Geometry check sheet. Reference: the model listing, model coordinates, mm. Round coordinates to 2 decimals unless told otherwise and drop trailing zeros. Write each loop counter-clockwise with the first axis right and the second up, starting at its lowest first coordinate (ties: lowest second). Pieces come first, ordered by that corner, then holes. Notation, with made-up numbers: M 48.25,13.5 L 72.25,13.5 A20 ccw 72.25,45.5 Z; hole C -11.75,-33.5 d2. An arc over 180 degrees is marked long. One line per item, written item: value. Start each with the question number.
1. Section check C-C (x = 3). Record the boundary of the cut face in (y, z) (1 decimal), and give its area (3 significant figures).
2. Scan lines: probe 1 along X at (y, z) = (45, 0.75); probe 2 along X at (y, z) = (49, 4.25); probe 3 along X at (y, z) = (32, -2). Record each from-to range of solid material in increasing order. Write a range as [from, to].
3. Section check A-A (z = 0.5). Record the boundary of the cut face in (x, y) (1 decimal).
4. Section check B-B (y = -1.5). Record the boundary of the cut face in (x, z), and give its area (3 significant figures).
5. Depth check by flat-ended pin: P1, Ø1.8, axis at x = -3.18, y = 49.21, coming from the -Z side; P2, Ø1, axis at x = -2.5, y = 0.5, coming from the +Z side; P3, Ø1.6, axis at x = 3, y = -10, coming from the -Z side. Enter the tip coordinate at first touch or a pass-through.
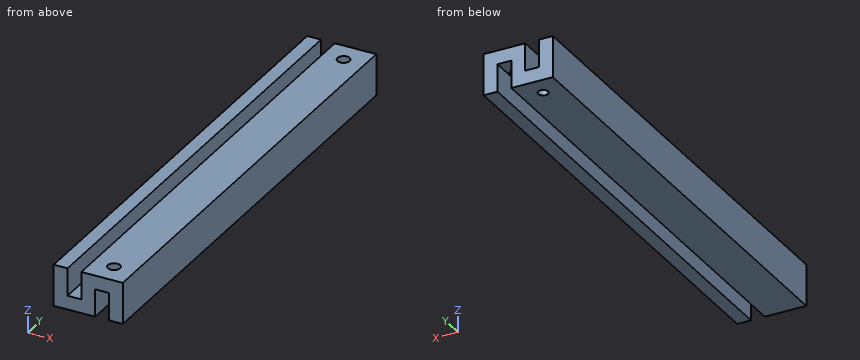
from build123d import *

# Parameters (mm, degrees)
EXTRUDE1_DEPTH                  = 53.975
SKETCH2_R                       = 1.1303
EXTRUDE2_DEPTH                  = 10.525
EXTRUDE3_REACH                  = 11.525
SKETCH3_R                       = 1.1303
F_4_40_TAPPED_HOLE1_D           = 2.2606
F_4_40_TAPPED_HOLE1_DEPTH       = 8.89
F_4_40_TAPPED_HOLE1_CBORE_D     = 2.8448
F_4_40_TAPPED_HOLE1_CBORE_DEPTH = 5.588
F_4_40_TAPPED_HOLE1_TIP         = 0.679152758


with BuildPart() as part:
    # Sketch1 → Extrude1 (new body, symmetric)
    with BuildSketch(Plane(origin=(0, 0, 0), x_dir=(1, 0, 0), z_dir=(0, 1, 0))):
        Polygon((-1.5875, -4.7625), (7.9375, -4.7625), (7.9375, 4.7625), (4.7625, 4.7625), (4.7625, -1.5875), (1.5875, -1.5875), (1.5875, 4.7625), (-7.9375, 4.7625), (-7.9375, -4.7625), (-4.7625, -4.7625), (-4.7625, 1.5875), (-1.5875, 1.5875), align=None)
    extrude(amount=EXTRUDE1_DEPTH, both=True)

    # Sketch2 → Extrude2 (cut, through all)
    with BuildSketch(Plane.XY.offset(4.7625)):
        with Locations((3.175, -48.895)):
            Circle(SKETCH2_R)
        with Locations((3.175, 48.895)):
            Circle(SKETCH2_R)
    extrude(amount=-EXTRUDE2_DEPTH, mode=Mode.SUBTRACT)

    # Sketch3 → Extrude3 (cut, up to next)
    with BuildSketch(Plane(origin=(0, 0, -4.7625), x_dir=(-1, 0, 0), z_dir=(0, 0, -1)), mode=Mode.PRIVATE) as extrude3_sk1:
        with Locations((3.175, 49.2125)):
            Circle(SKETCH3_R)
    extrude3_tool1 = extrude(extrude3_sk1.sketch, amount=-EXTRUDE3_REACH, mode=Mode.PRIVATE) & part.part
    add(extrude3_tool1.solids().sort_by_distance((-3.175, 49.2125, -4.7625))[0], mode=Mode.SUBTRACT)

    # #4-40 Tapped Hole1
    with Locations(Plane(origin=(3.175, 48.895, 4.7625), x_dir=(1, 0, 0), z_dir=(0, 0, 1))):
        with Locations((0, 0), (0, -97.79)):
            CounterBoreHole(F_4_40_TAPPED_HOLE1_D / 2, F_4_40_TAPPED_HOLE1_CBORE_D / 2, F_4_40_TAPPED_HOLE1_CBORE_DEPTH, depth=F_4_40_TAPPED_HOLE1_DEPTH)
            with Locations((0, 0, -(F_4_40_TAPPED_HOLE1_DEPTH + F_4_40_TAPPED_HOLE1_TIP / 2))):  # 118° drill point
                Cone(0, F_4_40_TAPPED_HOLE1_D / 2, F_4_40_TAPPED_HOLE1_TIP, mode=Mode.SUBTRACT)


solid = part.part
Result sheet:
1. outline: M -54,1.6 L -50.3,1.6 L -50.3,4.8 L -54,4.8 Z; M -47.5,1.6 L 47.5,1.6 L 47.5,4.8 L -47.5,4.8 Z; M 50.3,1.6 L 54,1.6 L 54,4.8 L 50.3,4.8 Z
1. area: 325 mm2
2. probe 1: x = [-7.94, -4.76], [-1.59, 1.59], [4.76, 7.94]
2. probe 2: x = [-7.94, -4.76], [-1.59, 1.76], [4.59, 7.94]
2. probe 3: x = [-7.94, 1.59], [4.76, 7.94]
3. outline: M -7.9,-54 L -4.8,-54 L -4.8,54 L -7.9,54 Z; M -1.6,-54 L 1.6,-54 L 1.6,54 L -1.6,54 Z; M 4.8,-54 L 7.9,-54 L 7.9,54 L 4.8,54 Z
4. outline: M -7.94,-4.76 L 1.59,-4.76 L 1.59,1.59 L 4.76,1.59 L 4.76,-4.76 L 7.94,-4.76 L 7.94,4.76 L -1.59,4.76 L -1.59,-1.59 L -4.76,-1.59 L -4.76,4.76 L -7.94,4.76 Z
4. area: 111 mm2
5. P1: passes through
5. P2: stops at z = -1.59
5. P3: stops at z = 1.59
